Autodesk Inventor part; units mm, degrees
ref_plane "YZ Plane" through (0, 0, 0) normal (1, 0, 0) x (0, 1, 0)
ref_plane "XZ Plane" through (0, 0, 0) normal (0, 1, 0) x (-1, 0, 0)
ref_plane "XY Plane" through (0, 0, 0) normal (0, 0, 1) x (1, 0, 0)
sketch "Skizze1" plane through (0, 0, 0) normal (0, 0, 1) x (1, 0, 0)
  line L0 (0, 0) -> (0, 3.5)
  line L1 (0, 3.5) -> (8, 3.5)
  line L2 (8, 3.5) -> (8, 27.3)
  line L3 (8, 27.3) -> (27, 27.3)
  line L4 (27, 27.3) -> (27, 25.795)
  line L5 (27, 25.795) -> (33, 25.795)
  line L6 (33, 25.795) -> (33, 19.795)
  line L7 (33, 19.795) -> (27, 19.795)
  line L8 (27, 19.795) -> (27, 17.795)
  line L9 (27, 17.795) -> (25, 12.3)
  line L10 (25, 12.3) -> (20, 12.3)
  line L11 (20, 12.3) -> (20, 11.5)
  line L12 (20, 11.5) -> (29.5, 11.5)
  line L13 (29.5, 11.5) -> (29.5, 3.5)
  line L14 (29.5, 3.5) -> (37.5, 3.5)
  line L15 (37.5, 3.5) -> (37.5, 0)
  line L16 (37.5, 0) -> (0, 0)
  line L17 (0, 32.76) -> (0, -5.46)
  line L18 (-7.5, 0) -> (45, 0)
  dimension "d0" = 27.3
  dimension "d1" = 3.5
  dimension "d2" = 37.5
  dimension "d3" = 8
  dimension "d4" = 19
  dimension "d5" = 6
  dimension "d6" = 6
  dimension "d7" = 15
  dimension "d8" = 11.5
  dimension "d9" = 21.5
  dimension "d10" = 12
  dimension "d11" = 17
  dimension "d12" = 2
  dimension "d13" = 70
extrude "Extrusion1" add sketch "Skizze1" along normal blind 10
sketch "Skizze2" plane through (0, 0, 0) normal (0, -1, 0) x (1, 0, 0)
  line L0 (37.5, 10) -> (0, 10)
  line L1 (37.5, 0) -> (37.5, 10)
  point P0 (25, 5)
  point P1 (17, 5)
  point P2 (21, 5)
  dimension "d16" = 16.5
  dimension "d17" = 4
  dimension "d18" = 4
  dimension "d19" = 5
  dimension "d20" = 5
  dimension "d21" = 5
hole "Bohrung1" at (25, 0, 5) at (17, 0, 5) at (21, 0, 5) direction (0, 1, 0) diameter 1.8 depth 3 tip angle 118
sketch "Skizze3" plane through (0, 0, 0) normal (0, -1, 0) x (1, 0, 0)
  circle A0 centre (21, 5) radius 0.9
  line L0 (37.5, 10) -> (0, 10)
  point P0 (33.5, 5)
  point P1 (4, 5)
  dimension "d30" = 12.5
  dimension "d31" = 17
  dimension "d32" = 5
  dimension "d33" = 5
hole "Bohrung2" at (33.5, 0, 5) at (4, 0, 5) direction (0, 1, 0) diameter 3.2 depth 3.5 tip angle 118
properties part number "Ventil" material "Thermoplastic Resin"
Model file for the job. Use its own axes, mm. A direction names the side the tool comes from. Round coordinates to 2 decimals unless told otherwise and drop trailing zeros. Loops run counter-clockwise (first coordinate to the right, second up) from the corner with the lowest first, then second, coordinate; pieces in that order, holes last. Notation, with made-up numbers: M 56,37 L 86,37 A13 ccw 86,62 Z; hole C -7,-39 d7. An arc over 180 degrees is marked long. Put each result on its own line as item: value. Start each with the question number.
Item 1: Cut at D-D (x = 6.5). List the corners of the cut face in (y, z).
Item 2: Cut at C-C (y = 21.75). List the corners of the cut face in (x, z), then the cut area to 3 significant figures.
Item 3: Mould opens along Y. For faces 1 (the face through (17, 27.3, 5)), 2 (the face through (24.11, 1.52, 5.12)), 3 (the face through (26.014, 15.086, 4.93)), 4 (the face through (25, 11.5, 5)) say: released by +Y, released by -Y, zero draft, split by the parting line, or undercut.
Item 4: Drill centre lines: line 1 along X through (y, z) = (2.3, 5); line 2 along Y through (x, z) = (22.5, 3); line 3 along Z through (x, y) = (33.5, 1.55). Where is each one in solid material? Low to high.
Item 5: 3-axis set-ups, long thin cutter, end or side, ignore diameter. For faces 5 (the face through (31.7, 3.5, 4.9)), 6 (the face through (27, 27, 5)), 7 (the face through (34.92, 1.77, 4.26)), 8 (the face through (6, 3.5, 5)): which of +Z, -Z, +X, -X, +Y, -Y reach the whole face in a straight line?
Item 6: Cut at A-A (x = 33.5). List the corners of the cut face in (y, z).
Item 7: Cut at B-B (z = 8.25). List the corners of the cut face in (x, y) (3 decimals).
Item 8: Drop flat-ended pins along their axis: P1, Ø4, axis at x = 2.5, z = 5, coming from the +Y side; P2, Ø0.9, axis at y = 11.5, z = 3, coming from the +X side; P3, Ø1.2, axis at y = 26.5, z = 4, coming from the +X side. Give the stop position or say it passes through.
Answer block:
1. outline: M 0,0 L 3.5,0 L 3.5,10 L 0,10 Z
2. outline: M 8,0 L 33,0 L 33,10 L 8,10 Z
2. area: 250 mm2
3. face 1: released by +Y
3. face 2: zero draft
3. face 3: undercut
3. face 4: undercut
4. line 1: 0 to 2.4, 5.6 to 16.1, 17.9 to 20.1, 21.9 to 24.1, 25.9 to 31.9, 35.1 to 37.5
4. line 2: 0 to 11.5, 12.3 to 27.3
4. line 3: 0 to 3.4, 6.6 to 10
5. face 5: +Z, -Z, +X
5. face 6: +Z, -Z, +X, +Y
5. face 7: -Y
5. face 8: +Z, -Z, -X, +Y
6. outline: M 0,0 L 3.5,0 L 3.5,3.4 L 0,3.4 Z; M 0,6.6 L 3.5,6.6 L 3.5,10 L 0,10 Z
7. outline: M 0,0 L 37.5,0 L 37.5,3.5 L 29.5,3.5 L 29.5,11.5 L 20,11.5 L 20,12.3 L 25,12.3 L 27,17.795 L 27,19.795 L 33,19.795 L 33,25.795 L 27,25.795 L 27,27.3 L 8,27.3 L 8,3.5 L 0,3.5 Z
8. P1: y = 3.5
8. P2: x = 29.5
8. P3: x = 27
